Can you work these out from the model? Positions are in its coordinate system, mm. A direction names the side the tool comes from. Give positions to 0.01 mm unless a question says otherwise; leave off trailing zeros. Write each loop counter-clockwise with the first axis right and the second up, starting at its lowest first coordinate (ties: lowest second). Pieces come first, ordered by that corner, then holes.
from build123d import *

# Parameters (mm, degrees)
SKETCH2_W                = 100
SKETCH2_H                = 100
BOSS_EXTRUDE1_DEPTH      = 3
SKETCH8_R                = 3
BOSS_EXTRUDE2_DEPTH      = 15.1
M3_CLEARANCE_HOLE1_D     = 3.2
F_4_0_4_DIAMETER_HOLE1_D = 4


with BuildPart() as part:
    # Sketch2 → Boss-Extrude1 (new body)
    with BuildSketch(Plane(origin=(0, 0, 0), x_dir=(1, 0, 0), z_dir=(0, 1, 0))):
        Rectangle(SKETCH2_W, SKETCH2_H)
    extrude(amount=BOSS_EXTRUDE1_DEPTH)

    # Sketch8 → Boss-Extrude2 (add)
    with BuildSketch(Plane.XZ):
        with Locations(Location((-11, -19.5, 0), (0, 0, 90))):
            Circle(SKETCH8_R)
        with Locations(Location((4, -19.5, 0), (0, 0, 90))):
            Circle(SKETCH8_R)
        with Locations(Location((4, -39.5, 0), (0, 0, 90))):
            Circle(SKETCH8_R)
        with Locations(Location((-11, -39.5, 0), (0, 0, 90))):
            Circle(SKETCH8_R)
    extrude(amount=BOSS_EXTRUDE2_DEPTH)

    # M3 Clearance Hole1 (through all)
    with Locations(Plane(origin=(0, 3, 0), x_dir=(1, 0, 0), z_dir=(0, 1, 0))):
        with Locations((-11, 39.5), (4, 39.5), (4, 19.5), (-11, 19.5), (19.5, 4), (39.5, 4), (39.5, -11), (19.5, -11)):
            Hole(M3_CLEARANCE_HOLE1_D / 2)

    # Ø4.0 (4) Diameter Hole1 (through all)
    with Locations(Plane(origin=(0, 3, 0), x_dir=(1, 0, 0), z_dir=(0, 1, 0))):
        with Locations((0, 0)):
            Hole(F_4_0_4_DIAMETER_HOLE1_D / 2)


solid = part.part
(1) Imagine slicing it at D-D, the plane x = 4. Write out the boundary of the cut face in (y, z).
Returned:
outline: (-15.1, -42.5) - (0, -42.5) - (0, -50) - (3, -50) - (3, -41.1) - (-15.1, -41.1) - close; (-15.1, -37.9) - (3, -37.9) - (3, -21.1) - (-15.1, -21.1) - (-15.1, -22.5) - (0, -22.5) - (0, -36.5) - (-15.1, -36.5) - close; (-15.1, -17.9) - (3, -17.9) - (3, 50) - (0, 50) - (0, -16.5) - (-15.1, -16.5) - close
(2) If I drill on L1, parallel to Z at x = 19.5, y = 1.1; L2, parallel to Z at x = -11, y = -10; L3, parallel to X at y = -8.5, z = -39.5, over which ranges is the centre line in solid material (lowest first)?
Returned:
L1: z = -50 to -5.6, -2.4 to 9.4, 12.6 to 50
L2: z = -42.5 to -41.1, -37.9 to -36.5, -22.5 to -21.1, -17.9 to -16.5
L3: x = -14 to -12.6, -9.4 to -8, 1 to 2.4, 5.6 to 7
(3) Imagine slicing it at C-C, the plane z = -19.5. Write out the boundary of the cut face in (x, y).
Returned:
outline: (-50, 0) - (-14, 0) - (-14, -15.1) - (-12.6, -15.1) - (-12.6, 3) - (-50, 3) - close; (-9.4, -15.1) - (-8, -15.1) - (-8, 0) - (1, 0) - (1, -15.1) - (2.4, -15.1) - (2.4, 3) - (-9.4, 3) - close; (5.6, -15.1) - (7, -15.1) - (7, 0) - (50, 0) - (50, 3) - (5.6, 3) - close
(4) Imagine slicing it at B-B, the plane x = 39.5. Write out the boundary of the cut face in (y, z).
Returned:
outline: (0, -50) - (3, -50) - (3, -5.6) - (0, -5.6) - close; (0, -2.4) - (3, -2.4) - (3, 9.4) - (0, 9.4) - close; (0, 12.6) - (3, 12.6) - (3, 50) - (0, 50) - close
(5) Will these pins go through, and if not, where does the flat tip stop? P1, Ø1.9, axis at x = -11, z = -39.5, coming from the +Y side; P2, Ø6, axis at x = -29.5, z = -4.5, coming from the -Y side; P3, Ø8, axis at x = -17, y = -0.5, coming from the +Z side.
Returned:
P1: passes through
P2: stops at y = 0
P3: stops at z = 50
(6) If we mould it in two halves opening along X, with no side actions, what happens to faces 1 (the face through (3.9, -7.4, -22.5)), 2 (the face through (50, 1, 1)), 3 (the face through (-11.1, -7.4, -22.5)), 4 (the face through (5, -15.1, -38))? For each: +X half, -X half, draft (parallel to the pull), parting line (faces both ways), or undercut.
Returned:
face 1: undercut
face 2: +X half
face 3: undercut
face 4: draft
(7) Imagine slicing it at A-A, the plane y = -2. Write out the boundary of the cut face in (x, z).
Returned:
outline: circle Ø6 at (-11, -39.5); circle Ø6 at (-11, -19.5); circle Ø6 at (4, -39.5); circle Ø6 at (4, -19.5); hole circle Ø3.2 at (-11, -39.5); hole circle Ø3.2 at (-11, -19.5); hole circle Ø3.2 at (4, -39.5); hole circle Ø3.2 at (4, -19.5)
(8) For faces 5 (the face through (0, 1, 2)), 6 (the face through (-11.1, -7.4, -42.5)), which set-ups out of +Z, -Z, +X, -X, +Y, -Y let a thin tool reach every point of the face, with its end or its side?
Returned:
face 5: +Y, -Y
face 6: -Y
